```python
from build123d import *

# Parameters (mm, degrees)
EXTRUDE009_DEPTH       = 500
SKETCH016_W            = 10
SKETCH016_H            = 10
EXTRUDE010_DEPTH       = 4
SKETCH019_R            = 3
EXTRUDE013_DEPTH       = 10.2
SKETCH013_R            = 10.75
SKETCH014_R            = 4.75
CUT008_PLACEMENT_ANGLE = 180


with BuildPart() as mast_slot_tool:
    # Sketch015 (on DatumPlane) → Extrude009 (new body)
    with BuildSketch(Plane(origin=(0, 8, 168), x_dir=(1, 0, 0), z_dir=(0, 0, 1))):
        with BuildLine():
            ThreePointArc((1.5, -8), (0, -6.5), (-1.5, -8))
            Line((-1.5, -8), (-1.5, -13))
            ThreePointArc((-1.5, -13), (0, -14.5), (1.5, -13))
            Line((1.5, -13), (1.5, -8))
        make_face()
    extrude(amount=-EXTRUDE009_DEPTH)


with BuildPart() as mast_zip_tool:
    # Sketch016 (on DatumPlane) → Extrude010 (new body)
    with BuildSketch(Plane.XY.offset(143)):
        with Locations((0, -5)):
            Rectangle(SKETCH016_W, SKETCH016_H)
        with Locations((0, 14.068966)):
            Rectangle(SKETCH016_W, SKETCH016_H)
    extrude(amount=EXTRUDE010_DEPTH)


with BuildPart() as upper_mast_hole:
    # Sketch019 (on DatumPlane) → Extrude013 (new body)
    with BuildSketch(Plane(origin=(0, 20, 23), x_dir=(1, 0, 0), z_dir=(0, 0, 1))):
        with Locations((0, -10.75)):
            Circle(SKETCH019_R)
    extrude(amount=EXTRUDE013_DEPTH)


with BuildPart() as upper_mast:
    # Sketch013 (on DatumPlane) → Loft section 0
    with BuildSketch(Plane(origin=(0, 20, 23), x_dir=(1, 0, 0), z_dir=(0, 0, 1))):
        with Locations((0, -10.75)):
            Circle(SKETCH013_R)
    # Sketch014 (on DatumPlane) → Loft section 1
    with BuildSketch(Plane(origin=(0, 8, 168), x_dir=(1, 0, 0), z_dir=(0, 0, 1))):
        with Locations((0, -4.75)):
            Circle(SKETCH014_R)
    loft()

    # Cut007: cut upper mast hole
    add(upper_mast_hole.part, mode=Mode.SUBTRACT)

    # Cut009: cut mast zip tool
    add(mast_zip_tool.part, mode=Mode.SUBTRACT)

    # Cut008: cut mast slot tool
    add(mast_slot_tool.part, mode=Mode.SUBTRACT)


with BuildPart() as upper_mast_1:
    # Cut008 placement: moved
    add(upper_mast.part.rotate(Axis((0, 0, 0), (0, 0, 1)), CUT008_PLACEMENT_ANGLE))


solid = upper_mast_1.part
```
For this review, take the finished solid that the model builds, in its own axes (mm). A direction names the side the tool comes from. Coordinates: 2 decimals unless noted, no trailing zeros. Use one line per item in the form item = value. Start each with the question number.
1) Draft analysis for pull direction Z (two halves, no side actions). For faces 1 (the face through (2.997, -9.382, 28.029)), 2 (the face through (-3, 0, 145)), 3 (the face through (0, -3, 168)), 4 (the face through (0, -9, 33.2)), state which applies: released by +Z, released by -Z, zero draft, split by the parting line, or undercut.
2) For pin 1 (4.5 mm diameter, centred on x = -1, z = 146, fed in from -Y); pin 2 (3 mm diameter, centred on x = 1, y = -8.5, fed in from -Z); pin 3 (1.9 mm diameter, centred on x = 2.5, z = 144.5, fed in from +Y), all flat-tipped, find the tip position at first contact; note any pin that passes through.
3) To check wall thickness, follow probe 1 along Y at (x, z) = (0, 28); probe 2 along X at (y, z) = (-9.25, 30.25); probe 3 along X at (y, z) = (-1, 69.5). State the ranges of each line that lie inside material, in increasing order. Write a range as from..to.
4) For faces 5 (the face through (0, -1.5, 96.5)), 6 (the face through (0, -9.069, 145)), 7 (the face through (3, 0, 145)), list the 3-axis set-ups (+Z, -Z, +X, -X, +Y, -Y) from which the entire face can be reached by the end or side of a thin tool; tool diameter is ignored.
From the geometry:
q1.face_1 = zero draft
q1.face_2 = undercut
q1.face_3 = released by +Z
q1.face_4 = released by -Z
q2.pin_1 = -9.74
q2.pin_2 = 33.2
q2.pin_3 = 0
q3.probe_1 = -19.59..-12.25, -6.25..-1.5
q3.probe_2 = -10.45..-3, 3..10.45
q3.probe_3 = -6.15..-1.12, 1.12..6.15
q4.face_5 = +Z, -Z, +Y
q4.face_6 = +X, -X, -Y
q4.face_7 = +X, -X, +Y
